Build history of the part. All positions in model axes, mm. Face numbers are marked on the shaded views. Round coordinates to 2 decimals unless told otherwise and drop trailing zeros. Write each loop counter-clockwise with the first axis right and the second up, starting at its lowest first coordinate (ties: lowest second). Pieces come first, ordered by that corner, then holes. Notation, with made-up numbers: (83, 75) -> (97, 75) arc R12 ccw to (97, 95) -> close; hole circle Ø11 at (86.25, -15). An arc over 180 degrees is marked (long way). Answer as CSV lines item,"result".
from build123d import *

# Parameters (mm, degrees)
F0_W      = 1200
F0_H      = 1000
F1_DEPTH  = 25
F2_W      = 1200
F2_H      = 100
F3_DEPTH  = 50
F4_W      = 1200
F4_H      = 100
F5_DEPTH  = 50
F6_R      = 20
F7_DEPTH  = 5
F8_W      = 50
F8_H      = 900
F9_DEPTH  = 100
F10_W     = 50
F10_H     = 900
F11_DEPTH = 100


with BuildPart() as f1:
    # F0 (on Front) → F1 (new body)
    with BuildSketch(Plane.XZ):
        Rectangle(F0_W, F0_H)
    extrude(amount=F1_DEPTH)

    # F2 (on face) → F3 (join)
    with BuildSketch(Plane.XY.offset(500)):
        with Locations((0, -75)):
            Rectangle(F2_W, F2_H)
    extrude(amount=-F3_DEPTH)

    # F4 (on face) → F5 (join)
    with BuildSketch(Plane(origin=(0, 0, -500), x_dir=(1, 0, 0), z_dir=(0, 0, -1))):
        with Locations((0, 75)):
            Rectangle(F4_W, F4_H)
    extrude(amount=-F5_DEPTH)

    # F6 (on face) → F7 (join)
    with BuildSketch(Plane.XZ.offset(125)):
        with Locations((-568, 475)):
            Circle(F6_R)
        with Locations((568, 475)):
            Circle(F6_R)
        with Locations((-568, -475)):
            Circle(F6_R)
        with Locations((568, -475)):
            Circle(F6_R)
    extrude(amount=F7_DEPTH)

    # F8 (on face) → F9 (join)
    with BuildSketch(Plane.XZ.offset(25)):
        with Locations((575, 0)):
            Rectangle(F8_W, F8_H)
    extrude(amount=F9_DEPTH)

    # F10 (on face) → F11 (join)
    with BuildSketch(Plane.XZ.offset(25)):
        with Locations((-575, 0)):
            Rectangle(F10_W, F10_H)
    extrude(amount=F11_DEPTH)


solid = f1.part
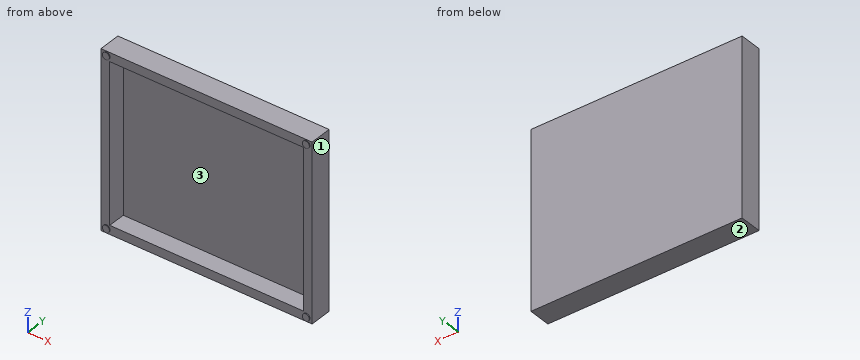
1. Drop a flat-ended pin along its axis: pin 1 Ø2 at (x, z) = (173.5, -78.5) entering from -Y. Give the stop position or say it passes through.
Results found:
pin 1,"stops at y = -25"
2. Mould opens along X. For the marked faces 1, 2 and 3 say: +X half, -X half, draft (parallel to the pull), parting line (faces both ways), or undercut.
Results found:
face 1,"+X half"
face 2,"draft"
face 3,"undercut"
3. Cut at B-B, the plane z = 350. Write the cut outline in (x, y).
Results found:
outline,"(-600, -125) -> (-550, -125) -> (-550, -25) -> (550, -25) -> (550, -125) -> (600, -125) -> (600, 0) -> (-600, 0) -> close"
4. Cut at D-D, the plane z = -475. Write the cut outline in (x, y).
Results found:
outline,"(-600, -125) -> (-588, -125) -> (-588, -130) -> (-548, -130) -> (-548, -125) -> (548, -125) -> (548, -130) -> (588, -130) -> (588, -125) -> (600, -125) -> (600, 0) -> (-600, 0) -> close"
5. Cut at A-A, the plane y = -105.5. Write the cut outline in (x, z), then the cut area to 3 significant figures.
Results found:
outline,"(-600, -500) -> (600, -500) -> (600, 500) -> (-600, 500) -> close; hole (-550, -450) -> (550, -450) -> (550, 450) -> (-550, 450) -> close"
area,"210,000 mm2"
6. Cut at C-C, the plane x = -568. Write the cut outline in (y, z), then the cut area to 3 significant figures.
Results found:
outline,"(-130, -495) -> (-125, -495) -> (-125, -500) -> (0, -500) -> (0, 500) -> (-125, 500) -> (-125, 495) -> (-130, 495) -> (-130, 455) -> (-125, 455) -> (-125, -455) -> (-130, -455) -> close"
area,"125,000 mm2"
7. Probe line 1 along Z through (x, y) = (522, -112.5); line 2 along X through (y, z) = (-84.5, 151.5); line 3 along Y through (x, z) = (-253, -191.5). List the from-to ranges inside material, lowest first.
Results found:
line 1,"z = -500 to -450, 450 to 500"
line 2,"x = -600 to -550, 550 to 600"
line 3,"y = -25 to 0"
